For this review, use the dimensioned drawing (mm, ordinates from the lowest corner) and the shaded views. A direction names the side the tool comes from. Round coordinates to 2 decimals unless told otherwise and drop trailing zeros. Loops run counter-clockwise (first coordinate to the right, second up) from the corner with the lowest first, then second, coordinate; pieces in that order, holes last. Notation, with made-up numbers: (79, 20.5) - (98, 20.5) arc R22 ccw to (98, 40.5) - close; hole circle Ø5 at (-25, -25). An arc over 180 degrees is marked (long way). Use one line per item in the form item = value. Start each with the question number.
(1) For pin 1 (1.5 mm diameter, centred on y = 4.5, z = 8.5, fed in from -X), flat-tipped, find the tip position at first contact; note if it passes through.
(2) Machinability: for the marked faces 1 and 2, which of the approach directions +Z, -Z, +X, -X, +Y, -Y give a long, thin tool a straight path to every point of the face, cutting with its end or side? Answer none if there is none.
(3) Wall thickness on probe 1 along Z at (x, y) = (3, 2.75); probe 2 along X at (y, z) = (2, 4) (1 decimal); probe 3 along X at (y, z) = (4.25, 10.5) (1 decimal): over which ranges is each line inside the solid? List them lowest first. Write a range as [from, to].
(4) We need section A-A, the plane z = 9.25. Write out the cut boundary in (x, y).
(5) We need section B-B, the plane y = 3.5. Write out the cut boundary in (x, z).
(6) We need section C-C, the plane x = 28.5. Write out the cut boundary in (y, z).
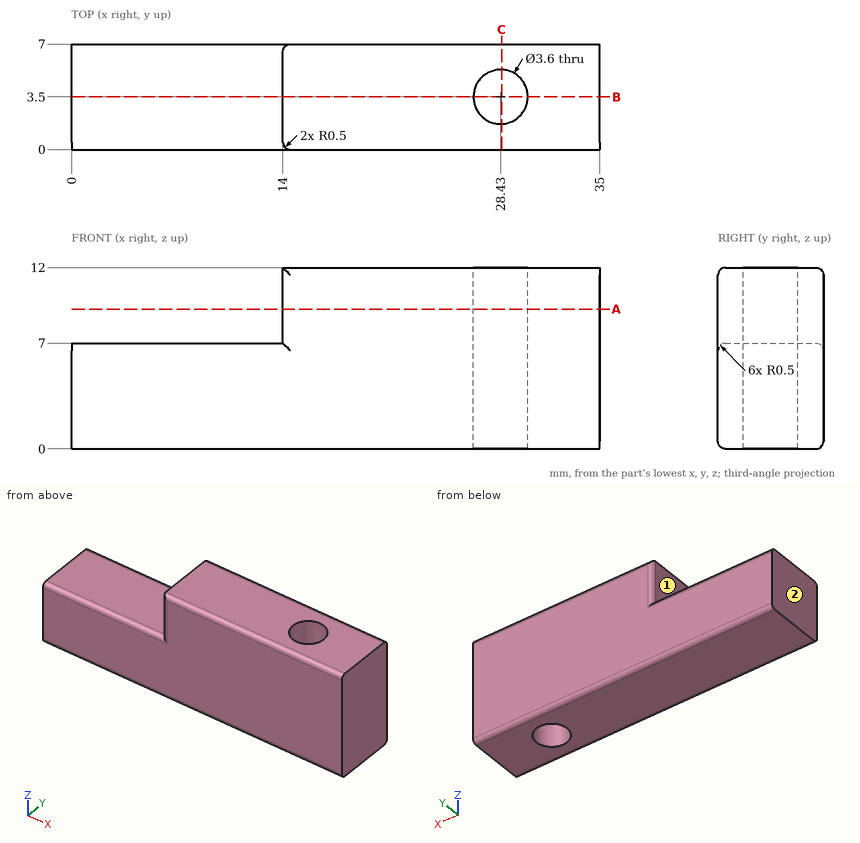
Data:
q1.pin_1 = 14
q2.face_1 = +Z, -X, +Y, -Y
q2.face_2 = +Z, -Z, -X, +Y, -Y
q3.probe_1 = [0, 7]
q3.probe_2 = [0, 27.4], [29.4, 35]
q3.probe_3 = [14, 26.8], [30.1, 35]
q4.outline = (14, 0.5) arc R0.5 ccw to (14.5, 0) - (35, 0) - (35, 7) - (14.5, 7) arc R0.5 ccw to (14, 6.5) - close; hole circle Ø3.6 at (28.43, 3.5)
q5.outline = (0, 0) - (26.63, 0) - (26.63, 12) - (14, 12) - (14, 7) - (0, 7) - close; (30.23, 0) - (35, 0) - (35, 12) - (30.23, 12) - close
q6.outline = (0, 0.5) arc R0.5 ccw to (0.5, 0) - (1.7, 0) - (1.7, 12) - (0.5, 12) arc R0.5 ccw to (0, 11.5) - close; (5.3, 0) - (6.5, 0) arc R0.5 ccw to (7, 0.5) - (7, 11.5) arc R0.5 ccw to (6.5, 12) - (5.3, 12) - close
